```python
from build123d import *

# Parameters (mm, degrees)
F1_DEPTH = 50.8
F2_R     = 3.175
F3_D     = 6.35
F3_DEPTH = 44.45
F3_TIP   = 1.9077324654


with BuildPart() as f1:
    # F0 (on Top) → F1 (new body)
    with BuildSketch(Plane.XY):
        with BuildLine():
            Line((6.35, -6.35), (6.35, 0))
            ThreePointArc((6.35, 0), (-4.4901280605, 4.4901280605), (0, -6.35))
            Line((0, -6.35), (6.35, -6.35))
        make_face()
    extrude(amount=F1_DEPTH)

    # F2
    f2_edges = [f1.edges().sort_by_distance(p)[0] for p in [
        (3.175, -6.35, 50.8),
        (6.35, -3.175, 50.8),
        (-4.490128, 4.490128, 50.8),
    ]]
    fillet(f2_edges, radius=F2_R)

    # F3
    with Locations(Plane(origin=(0, 0, 0), x_dir=(1, 0, 0), z_dir=(0, 0, -1))):
        with Locations((0, 0)):
            Hole(F3_D / 2, depth=F3_DEPTH)
            with Locations((0, 0, -(F3_DEPTH + F3_TIP / 2))):  # 118° drill point
                Cone(0, F3_D / 2, F3_TIP, mode=Mode.SUBTRACT)


solid = f1.part
```
Design review of the part built by this model. Coordinates are the model's own, in mm. Give positions to 0.01 mm unless a question says otherwise; leave off trailing zeros. Order: outer loops, then holes, each group sorted by start corner. A loop starts at its lowest first (then second) coordinate and runs counter-clockwise, first axis right, second up. Notation, with made-up numbers: M 21,52.5 L 38,52.5 A26 ccw 38,69.5 Z; hole C 33.25,59 d3. An arc over 180 degrees is marked long. One line per question, with ' | ' between items. Start each with the question number.
Q1. The part is to be moulded in two halves that separate along Y. For faces 1 (the face through (-0.072, -0.547, 46.026)), 2 (the face through (0.69, 3.1, 22.54)), 3 (the face through (0, 0, 50.8)), 4 (the face through (-4.34, 4.636, 23.479)), say which applies: +Y half, -Y half, draft (parallel to the pull), parting line (faces both ways), or undercut.
Q2. For pin 1 Ø1.5 at (x, y) = (1, 4.5) entering from +Z; pin 2 Ø1 at (x, z) = (-2, 44) entering from +Y; pin 3 Ø3 at (y, z) = (-4, 45) entering from -X, all flat-tipped, find the tip position at first contact; note any pin that passes through.
Q3. We need section A-A (z = 21). Write out the cut boundary in (x, y) (3 decimals), plus the area to 3 significant figures.
Q4. For L1, parallel to Y at x = 0.25, z = 40; L2, parallel to X at y = -2.25, z = 35.5; L3, parallel to Y at x = -1, z = 28.5, list the stretches that pass through material, from the lowest coordinate up. Write a range as [from, to].
Returned:
1) face 1: undercut | face 2: undercut | face 3: draft | face 4: parting line
2) pin 1: z = 50.73 | pin 2: y = 6.17 | pin 3: x = -5.84
3) outline: M 0,-6.35 L 6.35,-6.35 L 6.35,0 A6.35 ccw long Z; hole C 0,0 d6.35 | area: 104 mm2
4) L1: [-6.35, -3.17], [3.17, 6.35] | L2: [-5.94, -2.24], [2.24, 6.35] | L3: [-6.27, -3.01], [3.01, 6.27]
